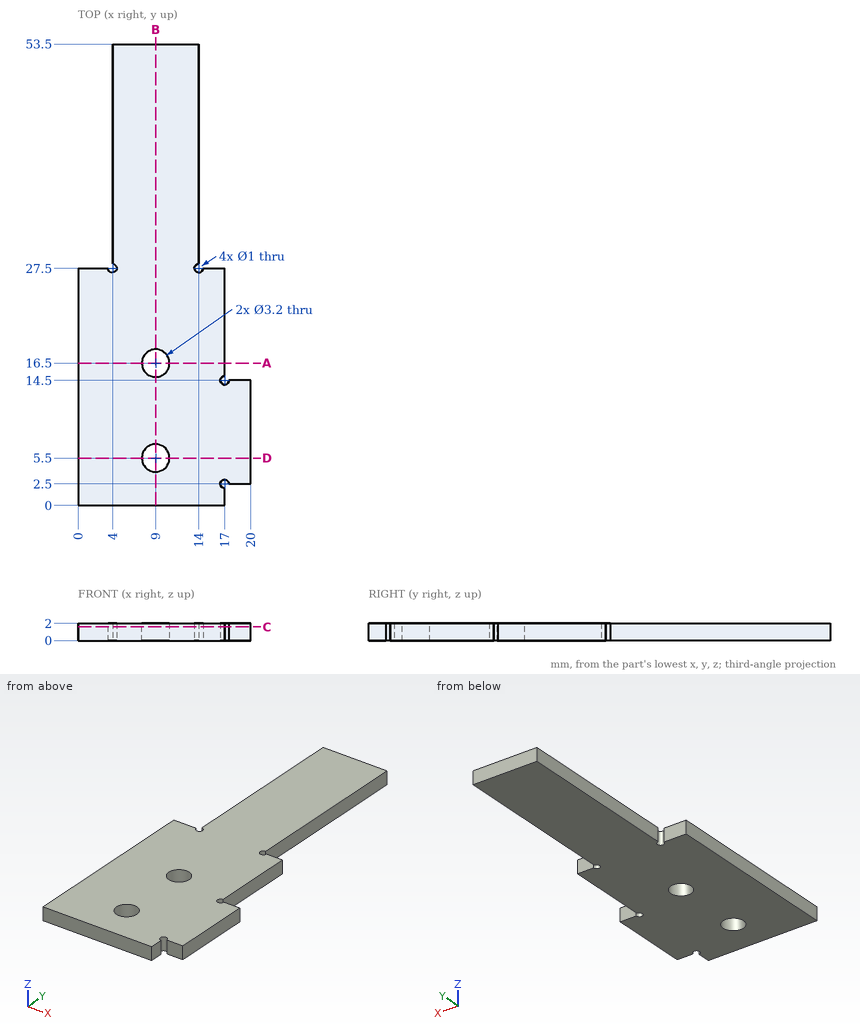
Print and shaded views of the part. All mm, measured from the part's lowest x, y and z. Coordinates: 2 decimals unless noted, no trailing zeros. Loops run counter-clockwise (first coordinate to the right, second up) from the corner with the lowest first, then second, coordinate; pieces in that order, holes last. Notation, with made-up numbers: (54, 12) - (103, 12) arc R34 ccw to (103, 44) - close; hole circle Ø6 at (85.25, 2). An arc over 180 degrees is marked (long way). Write item = value, one per line. Start each with the question number.
Item 1: Cut at B-B, the plane x = 9. Give the cut face in (y, z), and give its area (3 significant figures).
Item 2: Cut at A-A, the plane y = 16.5. Give the cut face in (x, z), and give its area (3 significant figures).
Item 3: Flat gauge pins, fed straight in: pin 1 Ø2.5 at (x, y) = (9, 5.5) entering from -Z; pin 2 Ø1 at (y, z) = (42, 1) entering from -X; pin 3 Ø1 at (x, z) = (15, 1) entering from +Y. Where does each tip first touch, or does it go through?
Item 4: Wall check: L1, parallel to Y at x = 9, z = 1.3; L2, parallel to X at y = 30.5, z = 0.2; L3, parallel to Y at x = 15.5, z = 0.6. Give the ranges that are in metal, low to high. Write a range as from..to.
Item 5: Cut at C-C, the plane z = 1.6. Give the cut face in (x, y), and give its area (3 significant figures).
Item 6: Cut at D-D, the plane y = 5.5. Give the cut face in (x, z).
The answers:
q1.outline = (0, 0) - (3.9, 0) - (3.9, 2) - (0, 2) - close; (7.1, 0) - (14.9, 0) - (14.9, 2) - (7.1, 2) - close; (18.1, 0) - (53.5, 0) - (53.5, 2) - (18.1, 2) - close
q1.area = 94.2 mm2
q2.outline = (0, 0) - (7.4, 0) - (7.4, 2) - (0, 2) - close; (10.6, 0) - (17, 0) - (17, 2) - (10.6, 2) - close
q2.area = 27.6 mm2
q3.pin_1 = through
q3.pin_2 = 4
q3.pin_3 = 27.5
q4.L1 = 0..3.9, 7.1..14.9, 18.1..53.5
q4.L2 = 4..14
q4.L3 = 0..27.5
q5.outline = (0, 0) - (17, 0) - (17, 2) arc R0.5 cw (long way) to (17.5, 2.5) - (20, 2.5) - (20, 14.5) - (17.5, 14.5) arc R0.5 cw (long way) to (17, 15) - (17, 27.5) - (14.5, 27.5) arc R0.5 cw (long way) to (14, 28) - (14, 53.5) - (4, 53.5) - (4, 28) arc R0.5 cw (long way) to (3.5, 27.5) - (0, 27.5) - close; hole circle Ø3.2 at (9, 5.5); hole circle Ø3.2 at (9, 16.5)
q5.area = 745 mm2
q6.outline = (0, 0) - (7.4, 0) - (7.4, 2) - (0, 2) - close; (10.6, 0) - (20, 0) - (20, 2) - (10.6, 2) - close
